```python
from build123d import *

# Parameters (mm, degrees)
BOSS_EXTRUDE1_DEPTH             = 94.9452
SKETCH2_R                       = 18.923
CUT_EXTRUDE1_DEPTH              = 56.9976
BOSS_EXTRUDE2_START             = -2.9972
BOSS_EXTRUDE2_DEPTH             = 2.9972
BOSS_EXTRUDE3_REACH             = 107.756
BOSS_EXTRUDE3_DIRECTION_2_REACH = 107.756
HOLE2_D                         = 7.9375
HOLE2_CBORE_D                   = 11.90625
HOLE2_CBORE_DEPTH               = 7.9375
CUT_EXTRUDE3_DEPTH              = 124.072551497
CUT_EXTRUDE3_DEPTH_BACK         = 124.072551497
SKETCH10_R                      = 3.96875
RIB1_REACH                      = 125.073
SKETCH11_WALL_W                 = 291.896910816
SKETCH11_WALL_H                 = 7.62
FILLET1_R                       = 2.54


with BuildPart() as part:
    # Sketch1 → Boss-Extrude1 (new body)
    with BuildSketch(Plane.XY):
        with BuildLine():
            Line((15.875, 0), (41.275, 0))
            Line((41.275, 0), (41.275, 21.59))
            Line((41.275, 21.59), (-41.275, 21.59))
            Line((-41.275, 21.59), (-41.275, 0))
            Line((-41.275, 0), (-15.875, 0))
            ThreePointArc((-15.875, 0), (0, 15.875), (15.875, 0))
        make_face()
    extrude(amount=BOSS_EXTRUDE1_DEPTH)

    # Sketch2 → Cut-Extrude1 (cut)
    with BuildSketch(Plane(origin=(0, 0, 0), x_dir=(-1, 0, 0), z_dir=(0, 0, -1))):
        Circle(SKETCH2_R)
    extrude(amount=-CUT_EXTRUDE1_DEPTH, mode=Mode.SUBTRACT)

    # Sketch3 → Boss-Extrude2 (add)
    with BuildSketch(Plane.XY.offset(94.9452).offset(BOSS_EXTRUDE2_START)):
        with BuildLine():
            Line((-9.017, 4.399409051), (-9.017, 0))
            Line((-9.017, 0), (-15.875, 0))
            ThreePointArc((-15.875, 0), (0, 15.875), (15.875, 0))
            Line((15.875, 0), (9.017, 0))
            Line((9.017, 0), (9.017, 4.399409051))
            ThreePointArc((9.017, 4.399409051), (0, 10.033), (-9.017, 4.399409051))
        make_face()
    extrude(amount=BOSS_EXTRUDE2_DEPTH)

    # Boss-Extrude3: up to this face of the body (flat: up to its plane)
    boss_extrude3_end = Plane(part.part.faces().sort_by_distance((41.275, 10.795, 47.4726))[0])
    # Sketch6 → Boss-Extrude3 (add, up to the picked face)
    with BuildSketch(Plane(origin=(0, 0, 0), x_dir=(0, 0, -1), z_dir=(1, 0, 0)), mode=Mode.PRIVATE) as boss_extrude3_sk1:
        Polygon((0, 21.59), (0, 66.548), (-21.59, 66.548), (-21.59, 60.198), (-12.7, 60.198), (-12.7, 21.59), align=None)
    boss_extrude3_tool1 = split(extrude(boss_extrude3_sk1.sketch, amount=BOSS_EXTRUDE3_REACH, mode=Mode.PRIVATE), bisect_by=boss_extrude3_end, keep=Keep.BOTH, mode=Mode.PRIVATE)
    # Sketch6 → Boss-Extrude3 (add, up to the picked face)
    with BuildSketch(Plane(origin=(0, 0, 0), x_dir=(0, 0, -1), z_dir=(1, 0, 0)), mode=Mode.PRIVATE) as boss_extrude3_sk2:
        Polygon((-51.308, 21.59), (-64.008, 21.59), (-64.008, 66.548), (-42.418, 66.548), (-42.418, 60.198), (-51.308, 60.198), align=None)
    boss_extrude3_tool2 = split(extrude(boss_extrude3_sk2.sketch, amount=BOSS_EXTRUDE3_REACH, mode=Mode.PRIVATE), bisect_by=boss_extrude3_end, keep=Keep.BOTH, mode=Mode.PRIVATE)
    add(boss_extrude3_tool1.solids().sort_by(Axis((0, 45.805864, 7.321272), (1, 0, 0)))[0])
    add(boss_extrude3_tool2.solids().sort_by(Axis((0, 45.805864, 56.686728), (1, 0, 0)))[0])

    # Boss-Extrude3 direction 2: up to this face of the body (flat: up to its plane)
    boss_extrude3_direction_2_end = Plane(part.part.faces().sort_by_distance((-41.275, 10.795, 47.4726))[0])
    # Sketch6 → Boss-Extrude3 direction 2 (add, up to the picked face)
    with BuildSketch(Plane(origin=(0, 0, 0), x_dir=(0, 0, -1), z_dir=(1, 0, 0)), mode=Mode.PRIVATE) as boss_extrude3_direction_2_sk1:
        Polygon((0, 21.59), (0, 66.548), (-21.59, 66.548), (-21.59, 60.198), (-12.7, 60.198), (-12.7, 21.59), align=None)
    boss_extrude3_direction_2_tool1 = split(extrude(boss_extrude3_direction_2_sk1.sketch, amount=-BOSS_EXTRUDE3_DIRECTION_2_REACH, mode=Mode.PRIVATE), bisect_by=boss_extrude3_direction_2_end, keep=Keep.BOTH, mode=Mode.PRIVATE)
    # Sketch6 → Boss-Extrude3 direction 2 (add, up to the picked face)
    with BuildSketch(Plane(origin=(0, 0, 0), x_dir=(0, 0, -1), z_dir=(1, 0, 0)), mode=Mode.PRIVATE) as boss_extrude3_direction_2_sk2:
        Polygon((-51.308, 21.59), (-64.008, 21.59), (-64.008, 66.548), (-42.418, 66.548), (-42.418, 60.198), (-51.308, 60.198), align=None)
    boss_extrude3_direction_2_tool2 = split(extrude(boss_extrude3_direction_2_sk2.sketch, amount=-BOSS_EXTRUDE3_DIRECTION_2_REACH, mode=Mode.PRIVATE), bisect_by=boss_extrude3_direction_2_end, keep=Keep.BOTH, mode=Mode.PRIVATE)
    add(boss_extrude3_direction_2_tool1.solids().sort_by(Axis((0, 45.805864, 7.321272), (-1, 0, 0)))[0])
    add(boss_extrude3_direction_2_tool2.solids().sort_by(Axis((0, 45.805864, 56.686728), (-1, 0, 0)))[0])

    # Hole2 (through all)
    with Locations(Plane(origin=(0, 21.59, 0), x_dir=(1, 0, 0), z_dir=(0, 1, 0))):
        with Locations((-30.099, -32.004), (-30.099, -82.2452)):
            hole2 = CounterBoreHole(HOLE2_D / 2, HOLE2_CBORE_D / 2, HOLE2_CBORE_DEPTH)

    # Mirror2: Hole2 across plane
    add(hole2.mirror(Plane(origin=(0, 0, 0), x_dir=(0, 0, 1), z_dir=(1, 0, 0))), mode=Mode.SUBTRACT)

    # Sketch10 → Cut-Extrude3 (cut, two sides: drawn at the far end of the back side and taken through both)
    with BuildSketch(Plane.XY.offset(-CUT_EXTRUDE3_DEPTH_BACK)):
        with Locations((-19.05, 40.894)):
            Circle(SKETCH10_R)
        with Locations((19.05, 40.894)):
            Circle(SKETCH10_R)
    extrude(amount=CUT_EXTRUDE3_DEPTH + CUT_EXTRUDE3_DEPTH_BACK, mode=Mode.SUBTRACT)

    # Sketch11 wall → Rib1 (add, up to next)
    with BuildSketch(Plane(origin=(0, 37.0586, 79.4766), x_dir=(0, 0.707106781187, -0.707106781187), z_dir=(0, 0.707106781187, 0.707106781187)), mode=Mode.PRIVATE) as rib1_sk1:
        Rectangle(SKETCH11_WALL_W, SKETCH11_WALL_H)
    rib1_tool1 = extrude(rib1_sk1.sketch, amount=-RIB1_REACH, mode=Mode.PRIVATE) - part.part
    add(rib1_tool1.solids().sort_by_distance((0, 37.0586, 79.4766))[0])

    # Fillet1
    fillet1_edges = [part.edges().sort_by_distance(p)[0] for p in [
        (-22.5425, 21.59, 64.008),
        (0, 60.198, 12.7),
        (0, 60.198, 21.59),
        (0, 66.548, 21.59),
        (0, 66.548, 0),
        (0, 21.59, 12.7),
        (22.5425, 21.59, 64.008),
        (0, 66.548, 64.008),
        (0, 66.548, 42.418),
        (0, 60.198, 42.418),
        (0, 60.198, 51.308),
        (0, 21.59, 51.308),
    ]]
    fillet(fillet1_edges, radius=FILLET1_R)


solid = part.part
```
Geometry check sheet. Reference: the model listing, model coordinates, mm. A direction names the side the tool comes from. Coordinates: 2 decimals unless noted, no trailing zeros. Order: outer loops, then holes, each group sorted by start corner. A loop starts at its lowest first (then second) coordinate and runs counter-clockwise, first axis right, second up. Notation, with made-up numbers: M -31.75,70.5 L -27.75,70.5 A17 cw -27.75,76.5 Z; hole C -27.75,31 d7. An arc over 180 degrees is marked long. One line per question, with ' | ' between items. Start each with the question number.
Item 1: Draft check along Y on faces 1 (the cylindrical face through (-0.578, 60.962, 43.142)), 2 (the cylindrical face through (-27.352, 17.677, 87.527)), 3 (the flat face through (-26, 13.652, 33)). Enter one of: pulls with the +Y half, pulls with the -Y half, needs draft (parallel to the pull), parting line crosses it, or undercut.
Item 2: Cross-section at B-B on x = 0. Enter the section's corners in (y, z) (3 decimals), then the cut area to 3 significant figures.
Item 3: Cross-section at A-A on y = 31. Enter the section's corners in (x, z) (3 decimals).
Item 4: Material ranges on L1, parallel to X at y = 41, z = 11 (3 decimals); L2, parallel to Y at x = -19.05, z = 59; L3, parallel to Y at x = -30, z = 45, recorded low to high. Write a range as [from, to].
Item 5: Set-up check for faces 4 (the flat face through (26, 13.652, 33)), 5 (the cylindrical face through (-22.28, 22.354, 64.732)), 6 (the cylindrical face through (-0.58, 65.82, 43.18)): record each of +Z, -Z, +X, -X, +Y, -Y from which the full face is reachable in a straight line by a thin tool's end or side.
Item 6: Gauge pin test, flat ends, axial feed: pin 1 (14 mm diameter, centred on x = 13.5, z = 83.5, fed in from +Y); pin 2 (8 mm diameter, centred on x = 27, y = 34.5, fed in from +Z); pin 3 (2 mm diameter, centred on y = 38, z = 67.5, fed in from -X). Record the tip position at first contact, or that the pin passes through.
Item 7: Cross-section at D-D on x = -21.5. State how many separate pieces and enclosed holes the cut face has, then the cut area to 3 significant figures.
Item 8: Cross-section at C-C on z = 24. Enter the section's corners in (x, y) (3 decimals).
Findings:
1) face 1: undercut | face 2: needs draft | face 3: pulls with the +Y half
2) outline: M 10.033,91.948 L 15.875,91.948 L 15.875,56.998 L 18.923,56.998 L 18.923,0 L 64.008,0 A2.54 ccw 66.548,2.54 L 66.548,19.05 A2.54 ccw 64.008,21.59 L 62.738,21.59 A2.54 ccw 60.198,19.05 L 60.198,15.24 A2.54 cw 57.658,12.7 L 24.13,12.7 A2.54 cw 21.59,15.24 L 21.59,48.768 A2.54 cw 24.13,51.308 L 57.658,51.308 A2.54 cw 60.198,48.768 L 60.198,44.958 A2.54 ccw 62.738,42.418 L 64.008,42.418 A2.54 ccw 66.548,44.958 L 66.548,61.468 A2.54 ccw 64.008,64.008 L 52.527,64.008 L 21.59,94.945 L 10.033,94.945 Z | area: 2,120 mm²
3) outline: M -41.275,0 L 41.275,0 L 41.275,12.7 L -41.275,12.7 Z; M -41.275,51.308 L 41.275,51.308 L 41.275,64.008 L 3.81,64.008 L 3.81,85.535 L -3.81,85.535 L -3.81,64.008 L -41.275,64.008 Z
4) L1: x = [-41.275, -23.017], [-15.083, 15.083], [23.017, 41.275] | L2: y = [0, 36.93], [44.86, 66.55] | L3: y = [0, 21.59], [60.2, 66.55]
5) face 4: +Y | face 5: +Z, -X, +Y | face 6: +X, -X, +Y
6) pin 1: stops at y = 21.59 | pin 2: stops at z = 64.01 | pin 3: stops at x = -3.81
7) separate pieces: 3 | enclosed holes: 0 | area: 3,140 mm²
8) outline: M -41.275,0 L -18.923,0 A18.923 cw 18.923,0 L 41.275,0 L 41.275,21.59 L -41.275,21.59 Z
